Autodesk Inventor part; units mm, degrees
ref_plane "YZ Plane" through (0, 0, 0) normal (1, 0, 0) x (0, 1, 0)
ref_plane "XZ Plane" through (0, 0, 0) normal (0, 1, 0) x (-1, 0, 0)
ref_plane "XY Plane" through (0, 0, 0) normal (0, 0, 1) x (1, 0, 0)
sketch "Sketch1" plane through (0, 0, 0) normal (0, 1, 0) x (-1, 0, 0)
  line L0 (0, 0) -> (1, 0)
  line L1 (1, 0) -> (1, -8)
  line L2 (1, -8) -> (0, -8)
  line L3 (0, -8) -> (0, 0)
  line L4 (1, 0) -> (11.5, 0)
  line L5 (11.5, 0) -> (11.5, -14)
  line L6 (11.5, -14) -> (1, -14)
  line L7 (1, -14) -> (1, 0)
  line L8 (0, 0) -> (-13, 0)
  line L9 (-13, 0) -> (-13, -25)
  line L10 (-13, -25) -> (0, -25)
  line L11 (0, -25) -> (0, 0)
  line L12 (-13, -23) -> (0, -20.118)
  line L13 (-13, 0) -> (11.5, 0)
  line L14 (11.5, 0) -> (11.5, -25)
  line L15 (11.5, -25) -> (-13, -25)
  line L16 (-13, -25) -> (-13, 0)
  line L17 (-13, -25) -> (0, -22.118) construction
  line L18 (11.5, -25) -> (15.5, -25)
  line L19 (15.5, -25) -> (15.5, -18.5)
  line L20 (15.5, -18.5) -> (11.5, -18.5)
  line L21 (11.5, -18.5) -> (11.5, -25)
  line L22 (0, -8) -> (-5, -8)
  line L23 (-5, -8) -> (-5, -12)
  line L24 (-5, -12) -> (0, -12)
  line L25 (0, -12) -> (0, -8)
  line L26 (1, -8) -> (-2, -8)
  line L27 (-2, -8) -> (-2, -25)
  line L28 (-2, -25) -> (1, -25)
  line L29 (1, -25) -> (1, -8)
  line L30 (1, -25) -> (15.5, -21.7854)
  line L31 (-5, -8) -> (-4, -8)
  line L32 (-4, -8) -> (-4, -9.1)
  line L33 (-4, -9.1) -> (-5, -9.1)
  line L34 (-5, -9.1) -> (-5, -8)
  point P0 (1, -8)
  point P1 (0, -8)
  point P2 (0, -25)
  point P3 (11.5, -18.5)
  point P4 (0, -12)
  point P5 (0, -8)
  point P6 (0, -25)
  point P7 (-2, -12)
  point P8 (-2, -20.5614)
  point P9 (1, -25)
  dimension "d0" = 1
  dimension "d1" = 8
  dimension "d2" = 10.5
  dimension "d3" = 14
  dimension "d6" = 13
  dimension "d7" = 25
  dimension "d9" = 23
  dimension "d35" = 4
  dimension "d36" = 18.5
  dimension "d41" = 4
  dimension "d42" = 12.5
  dimension "d43" = 6
  dimension "d44" = 3
  dimension "d45" = 1
  dimension "d46" = 1.1
revolve "Revolution1" add sketch "Sketch1" angle 360 about axis through (0, 0, 0) along (-1, 0, 0) contours L2 L7 L29 L15 L11 | L11 L24 L27 L22 | L11 L12 L27 L24 | L27 L24 L23 L33 L32 L22 | L12 L27 L10 L9 | L6 L14 L30 L29 | L11 L10 L27 L12 | L20 L19 L30 L14
chamfer "Chamfer2" distance 0.5 angle 45 1 edges at (-1, 0, 8)
chamfer "Chamfer4" distance 0.5 angle 45 1 edges at (13, 0, 25)
chamfer "Chamfer5" distance 2 angle 45 1 edges at (-11.5, 0, 14)
properties part number "Flywheel" material "Brass, Soft Yellow"
Can you work these out from the model? Positions are in its coordinate system, mm. A direction names the side the tool comes from. Round coordinates to 2 decimals unless told otherwise and drop trailing zeros. Order: outer loops, then holes, each group sorted by start corner. A loop starts at its lowest first (then second) coordinate and runs counter-clockwise, first axis right, second up. Notation, with made-up numbers: M -7.75,-16.5 L 32.25,-16.5 A16 ccw 32.25,-6.5 Z; hole C -32,70 d3. An arc over 180 degrees is marked long. Use a Markdown table: item, result.
1) On a 3-axis mill with a long thin cutter (end or side, diameter ignored), from which of +Z, -Z, +X, -X, +Y, -Y can I reach the whole of each face in a straight line? I mean faces 1 (the face through (-11.5, -15, 6)), 2 (the face through (4, 7, -5)), 3 (the face through (1.78, -7.81, 1.73)). Say none if no direction works.
Geometry says:
| item | result |
|---|---|
| face 1 | -X |
| face 2 | +X |
| face 3 | +X, -X |
2) If we mould it in two halves opening along Y, with no side actions, what happens to faces 4 (the face through (5.656, -7.509, -23.846)), 5 (the face through (2, 9, -9)), 6 (the face through (-15.5, 16, 10))? For each: +Y half, -Y half, draft (parallel to the pull), parting line (faces both ways), or undercut.
Geometry says:
| item | result |
|---|---|
| face 4 | parting line |
| face 5 | undercut |
| face 6 | draft |
3) I'm going to push flat-ended pins straight in: P1, Ø16.5, axis at y = 0, z = 0, coming from the +X side; P2, Ø12, axis at x = 8, z = -9, coming from the +Y side; P3, Ø4, axis at x = 3.5, z = 15, coming from the +Y side; P4, Ø5, axis at y = -3.5, z = -1, coming from the +X side. Where does each tip first touch, or does it pass through?
Geometry says:
| item | result |
|---|---|
| P1 | stops at x = 4 |
| P2 | stops at y = 24.82 |
| P3 | stops at y = 21.35 |
| P4 | passes through |
4) Imagine slicing it at B-B (x = 10.25). List the corners of the cut face in (y, z) for me.
Geometry says:
| item | result |
|---|---|
| outline | C 0,0 d50; hole C 0,0 d44.78 |
5) If I drill on line 1 along Z through (x, y) = (4.75, -5); line 2 along Y through (x, z) = (4.3, 0); line 3 along Y through (x, z) = (0.8, 0), over which ranges is the centre line in solid material (lowest first)?
Geometry says:
| item | result |
|---|---|
| line 1 | z = -24.49 to -20.57, -10.91 to -7.6, 7.6 to 10.91, 20.57 to 24.49 |
| line 2 | y = -25 to -21.07, -12 to -9.1, 9.1 to 12, 21.07 to 25 |
| line 3 | y = -25 to -8, 8 to 25 |
6) Imagine slicing it at A-A (x = -5.75). List the corners of the cut face in (y, z) for me.
Geometry says:
| item | result |
|---|---|
| outline | C 0,0 d47.89; hole C 0,0 d28 |
